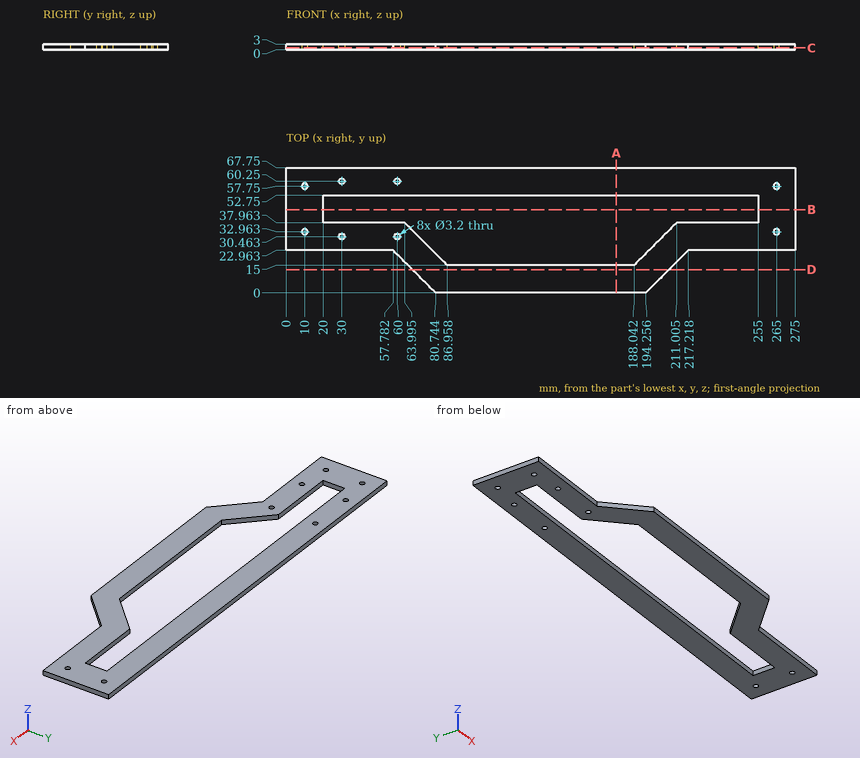
Design review of the part shown in the three views and the two pictorial views. Dimensions are in mm from the part's minimum x, y and z. Round coordinates to 2 decimals unless told otherwise and drop trailing zeros. Write each loop counter-clockwise with the first axis right and the second up, starting at its lowest first coordinate (ties: lowest second). Pieces come first, ordered by that corner, then holes.
Item 1: We need section C-C on z = 0.9. State how many separate pieces and enclosed holes the cut face has, and give its area (3 significant figures).
Item 2: We need section B-B on y = 45. Write out the cut boundary in (x, z), and give its area (3 significant figures).
Item 3: We need section D-D on y = 12.5. Write out the cut boundary in (x, z) (1 decimal).
Item 4: Clearance check with flat-ended pins moving along their axes: pin 1 Ø1.5 at (y, z) = (9, 0.5) entering from +X (1 decimal); pin 2 Ø1.5 at (x, z) = (25, 1) entering from -Y; pin 3 Ø1 at (y, z) = (7.5, 1) entering from +X (1 decimal). State where each tip first meets the part, or that it passes through.
Item 5: We need section A-A on x = 178.5. Write out the cut boundary in (y, z).
Item 6: For probe 1 along Y at (x, z) = (30, 1.2); probe 2 along X at (y, z) = (43, 0.8); probe 3 along Y at (x, z) = (50, 2.35), list the stretches that pass through material, from the lowest coordinate up.
Returned:
1. separate pieces: 1
1. enclosed holes: 9
1. area: 9,060 mm2
2. outline: (0, 0) - (20, 0) - (20, 3) - (0, 3) - close; (255, 0) - (275, 0) - (275, 3) - (255, 3) - close
2. area: 120 mm2
3. outline: (68.2, 0) - (206.8, 0) - (206.8, 3) - (68.2, 3) - close
4. pin 1: stops at x = 204
4. pin 2: stops at y = 22.96
4. pin 3: stops at x = 202.3
5. outline: (0, 0) - (15, 0) - (15, 3) - (0, 3) - close; (52.75, 0) - (67.75, 0) - (67.75, 3) - (52.75, 3) - close
6. probe 1: y = 22.96 to 28.86, 32.06 to 37.96, 52.75 to 58.65, 61.85 to 67.75
6. probe 2: x = 0 to 20, 255 to 275
6. probe 3: y = 22.96 to 37.96, 52.75 to 67.75
